The figure shows three views and two pictorial views of one solid part (mm, origin at its lowest corner). Answer the questions. A direction names the side the tool comes from. Coordinates: 2 decimals unless noted, no trailing zeros. Loops run counter-clockwise (first coordinate to the right, second up) from the corner with the lowest first, then second, coordinate; pieces in that order, holes last. Notation, with made-up numbers: (30.5, 25) - (60.5, 25) arc R26 cw to (60.5, 59) - close; hole circle Ø3 at (76, 36). An arc over 180 degrees is marked (long way). Write each question's results on one line, items separated by ' | '. Start each with the question number.
Item 1: A tool of negligible diameter and unlimited length cuts with its end or side. For the marked faces 1 and 2, from which of +Z, -Z, +X, -X, +Y, -Y can it reach the whole face along a straight path? Write none if from no direction.
Item 2: Section C-C, the plane y = 24.5 is taken. Write down the section's boundary in (x, z).
Item 3: Section B-B, the plane z = 22 is taken. Write down the section's boundary in (x, y).
Item 4: Section A-A, the plane x = 21 is taken. Write down the section's boundary in (y, z), plus the area to 3 significant figures.
Item 5: Consider probe 1 along Z at (x, y) = (19.75, 32.5); probe 2 along Y at (x, z) = (3.75, 22.5); probe 3 along Z at (x, y) = (3, 7.5). Determine where each line is inside the solid, lowest interval first. Write a range as [from, to].
Item 6: Each of these flat-tipped pins is pushed along its axis until it touches: pin 1 Ø7.5 at (x, z) = (13, 31.5) entering from +Y; pin 2 Ø5 at (x, y) = (13, 28) entering from -Z. Where does it stop, or does it pass through?
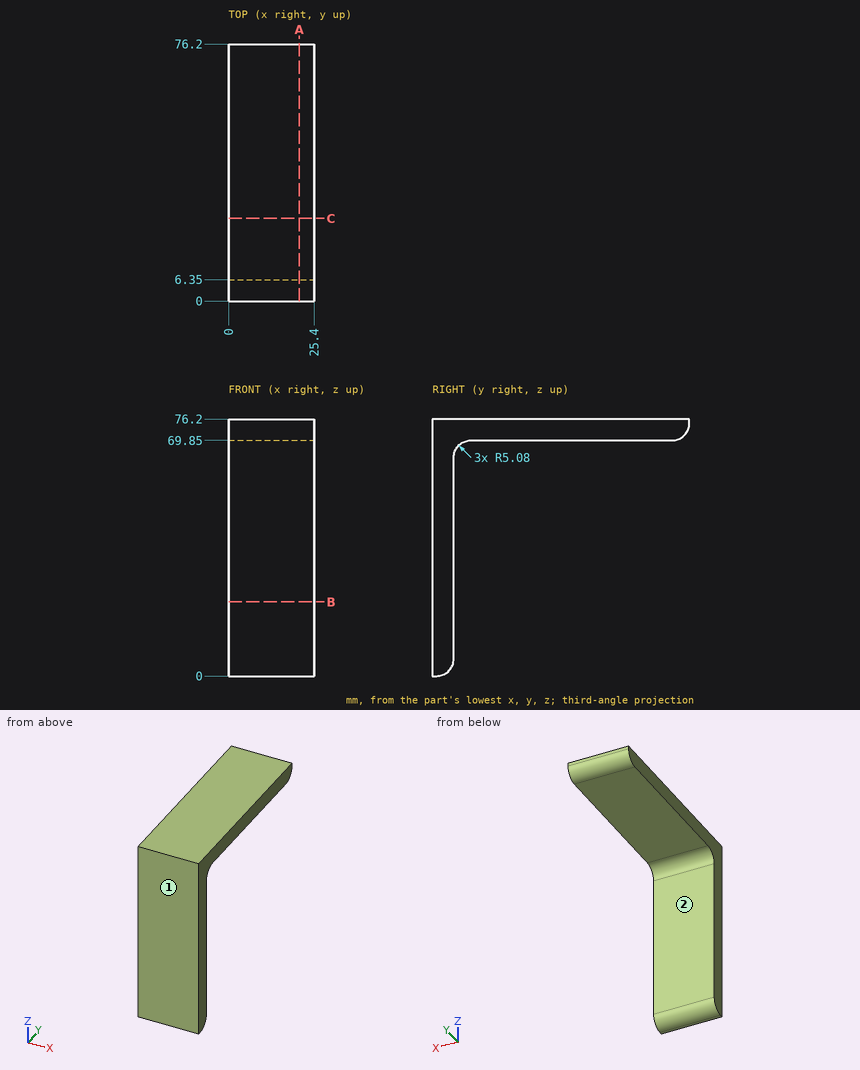
Answer key:
1) face 1: +Z, -Z, +X, -X, -Y | face 2: -Z, +X, -X, +Y
2) outline: (0, 69.85) - (25.4, 69.85) - (25.4, 76.2) - (0, 76.2) - close
3) outline: (0, 0) - (25.4, 0) - (25.4, 6.35) - (0, 6.35) - close
4) outline: (0, 0) - (1.27, 0) arc R5.08 ccw to (6.35, 5.08) - (6.35, 64.77) arc R5.08 cw to (11.43, 69.85) - (71.12, 69.85) arc R5.08 ccw to (76.2, 74.93) - (76.2, 76.2) - (0, 76.2) - close | area: 922 mm^2
5) probe 1: z = [69.85, 76.2] | probe 2: y = [0, 6.35] | probe 3: z = [67.99, 76.2]
6) pin 1: stops at y = 6.35 | pin 2: stops at z = 69.85
